```python
from build123d import *

# Parameters (mm, degrees)
F0_R     = 25
F0_R_2   = 23
F1_DEPTH = 25
F0_R_3   = 6.834856
F0_R_4   = 3.562232
F0_R_5   = 4.797994
F0_R_6   = 6.041215
F2_DEPTH = 5
F3_DEPTH = 25


with BuildPart() as f1:
    # F0 (on Top) → F1 (new body)
    with BuildSketch(Plane.XY):
        Circle(F0_R)
        Circle(F0_R_2, mode=Mode.SUBTRACT)
    extrude(amount=F1_DEPTH)

    # F0 (on Top) → F2 (join)
    with BuildSketch(Plane.XY):
        Circle(F0_R_2)
        with Locations((-8.042553, -7.707447)):
            Circle(F0_R_3, mode=Mode.SUBTRACT)
        with Locations((10.723404, -9.047872)):
            Circle(F0_R_4, mode=Mode.SUBTRACT)
        with Locations((-13.06915, 10.723405)):
            Circle(F0_R_5, mode=Mode.SUBTRACT)
        with Locations((6.031916, 11.058511)):
            Circle(F0_R_6, mode=Mode.SUBTRACT)
    extrude(amount=F2_DEPTH)

    # F0 (on Top) → F3 (join)
    with BuildSketch(Plane.XY):
        with Locations((-8.042553, -7.707447)):
            Circle(F0_R_3)
        with Locations((6.031916, 11.058511)):
            Circle(F0_R_6)
        with Locations((-13.06915, 10.723405)):
            Circle(F0_R_5)
        with Locations((10.723404, -9.047872)):
            Circle(F0_R_4)
    extrude(amount=F3_DEPTH)


solid = f1.part
```
Check sheet for the modelled part. Datum: model origin and axes. Units: mm. A direction names the side the tool comes from. Coordinates: 2 decimals unless noted, no trailing zeros. Order: outer loops, then holes, each group sorted by start corner. A loop starts at its lowest first (then second) coordinate and runs counter-clockwise, first axis right, second up. Notation, with made-up numbers: M 80,-27.5 L 131,-27.5 A17 cw 131,3.5 Z; hole C 82.5,57 d5. An arc over 180 degrees is marked long. Write each question's results on one line, items separated by ' | '. Start each with the question number.
1. Mould release check, pull along Y, two halves, no side actions. Record for faces 1 (the face through (0, 0, 5)), 2 (the face through (14.12, -7.98, 14.86)), 3 (the face through (23.846, 7.509, 12.325)), 4 (the face through (6, 11, 25)): +Y half, -Y half, draft (parallel to the pull), parting line (faces both ways), or undercut.
2. Go/stop test with flat-tipped pins: P1, Ø5, axis at x = -12, z = 8.5, coming from the -Y side; P2, Ø8, axis at x = 19.5, z = 19.5, coming from the -Y side; P3, Ø6, axis at x = 9, z = 2.5, coming from the +Y side. Record where each tip stops, or that it passes through.
3. Cross-section at D-D on y = 8. Record the cut outline in (x, z).
4. Cross-section at A-A on y = 0. Record the cut outline in (x, z).
5. Cross-section at B-B on x = -19.5. Record the cut outline in (y, z).
6. Material ranges on probe 1 along Y at (x, z) = (-14, 21); probe 2 along Y at (x, z) = (4, 19); probe 3 along Z at (x, y) = (18.5, 0), recorded low to high.
7. Cross-section at C-C on x = -6. Record the cut outline in (y, z).
8. Access from +Z, -Z, +X, -X, +Y, -Y to the whole of each face (thin tool, end or side, straight path). Record for faces 5 (the face through (1.58, 15.14, 14.86)), 6 (the face through (-8, -8, 25)).
Checks:
1) face 1: undercut | face 2: undercut | face 3: parting line | face 4: draft
2) P1: stops at y = -23.12 | P2: stops at y = -19.62 | P3: stops at y = 24.27
3) outline: M -23.69,0 L 23.69,0 L 23.69,25 L 21.56,25 L 21.56,5 L 11.24,5 L 11.24,25 L 0.82,25 L 0.82,5 L -9.12,5 L -9.12,25 L -17.02,25 L -17.02,5 L -21.56,5 L -21.56,25 L -23.69,25 Z
4) outline: M -25,0 L 25,0 L 25,25 L 23,25 L 23,5 L -23,5 L -23,25 L -25,25 Z
5) outline: M -15.64,0 L 15.64,0 L 15.64,25 L 12.2,25 L 12.2,5 L -12.2,5 L -12.2,25 L -15.64,25 Z
6) probe 1: y = -20.71 to -18.25, -11.06 to -4.36, 6.02 to 15.43, 18.25 to 20.71 | probe 2: y = -24.68 to -22.65, 5.37 to 16.75, 22.65 to 24.68 | probe 3: z = 0 to 5
7) outline: M -24.27,0 L 24.27,0 L 24.27,25 L 22.2,25 L 22.2,5 L -1.18,5 L -1.18,25 L -14.23,25 L -14.23,5 L -22.2,5 L -22.2,25 L -24.27,25 Z
8) face 5: +Z | face 6: +Z, +X, -X, +Y, -Y
